Build history of the part. All positions in model axes, mm. Give positions to 0.01 mm unless a question says otherwise; leave off trailing zeros. Loops run counter-clockwise (first coordinate to the right, second up) from the corner with the lowest first, then second, coordinate; pieces in that order, holes last. Notation, with made-up numbers: M -27.5,-10 L -6.5,-10 A14 cw -6.5,11 Z; hole C 12.5,-37.75 d7. An arc over 180 degrees is marked long. Answer as a JSON object with one key per item and string values. Group by question number.
1. Drill centre lines: line 1 along X through (y, z) = (-46.5, 1.75); line 2 along Y through (x, z) = (4, 1.1); line 3 along X through (y, z) = (-42, 1.05). Where is each one in solid material? Low to high. Write a range as [from, to].
2. Slice it at A-A (z = 0.9). List the corners of the cut face in (x, y), then the cut area to 3 significant figures.
3. Slice it at B-B (x = -23). List the corners of the cut face in (y, z), then the cut area to 3 significant figures.
from build123d import *

# Parameters (mm, degrees)
F0_W     = 76.2
F0_H     = 30.1752
F1_DEPTH = 2.4638
F2_R     = 3.81
F3_DEPTH = 20.32


with BuildPart() as f1:
    # F0 (on Top) → F1 (new body)
    with BuildSketch(Plane.XY):
        with Locations((-4.829727, -43.646489)):
            Rectangle(F0_W, F0_H)
    extrude(amount=F1_DEPTH)

    # F2 (on Top) → F3 (cut)
    with BuildSketch(Plane.XY):
        with Locations((-22.441126, -45.335913)):
            Circle(F2_R)
        with BuildLine():
            ThreePointArc((-8.594292, -50.796484), (-6.094356, -49.760976), (-5.058848, -47.26104))
            ThreePointArc((-5.058848, -47.26104), (-6.094356, -44.761104), (-8.594292, -43.725596))
            Line((-8.594292, -43.725596), (-8.594292, -50.796484))
        make_face()
        with BuildLine():
            Line((-8.594292, -50.796484), (-8.594292, -43.725596))
            ThreePointArc((-8.594292, -43.725596), (-12.129736, -47.26104), (-8.594292, -50.796484))
        make_face()
        with Locations((3.573384, -47.173662)):
            Circle(F2_R)
    extrude(amount=F3_DEPTH, mode=Mode.SUBTRACT)


solid = f1.part
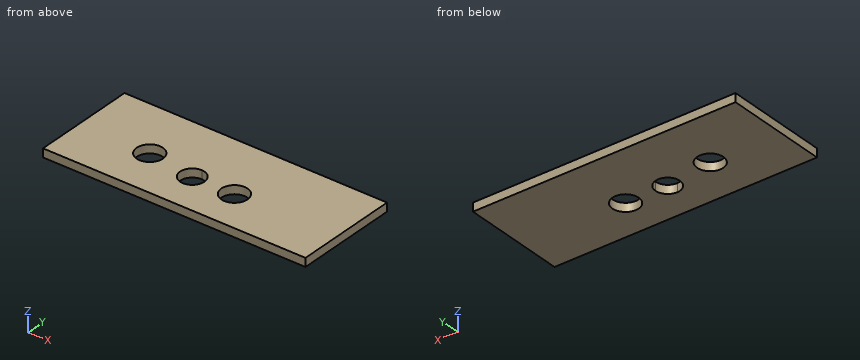
Established:
{
 "1": {"line 1": "x = [-42.93, -26.07], [-18.81, -12.05], [-5.14, -0.18], [7.32, 33.27]", "line 2": "y = [-58.73, -50.96], [-43.39, -28.56]", "line 3": "x = [-42.93, -24.28], [-20.6, 33.27]"},
 "2": {"outline": "M -42.93,-58.73 L 33.27,-58.73 L 33.27,-28.56 L -42.93,-28.56 Z; hole C -22.44,-45.34 d7.62; hole M -8.59,-50.8 A3.54 ccw -5.06,-47.26 A3.54 ccw -8.59,-43.73 A3.54 ccw Z; hole C 3.57,-47.17 d7.62", "area": "2,170 mm^2"},
 "3": {"outline": "M -58.73,0 L -49.1,0 L -49.1,2.46 L -58.73,2.46 Z; M -41.57,0 L -28.56,0 L -28.56,2.46 L -41.57,2.46 Z", "area": "55.8 mm^2"}
}
